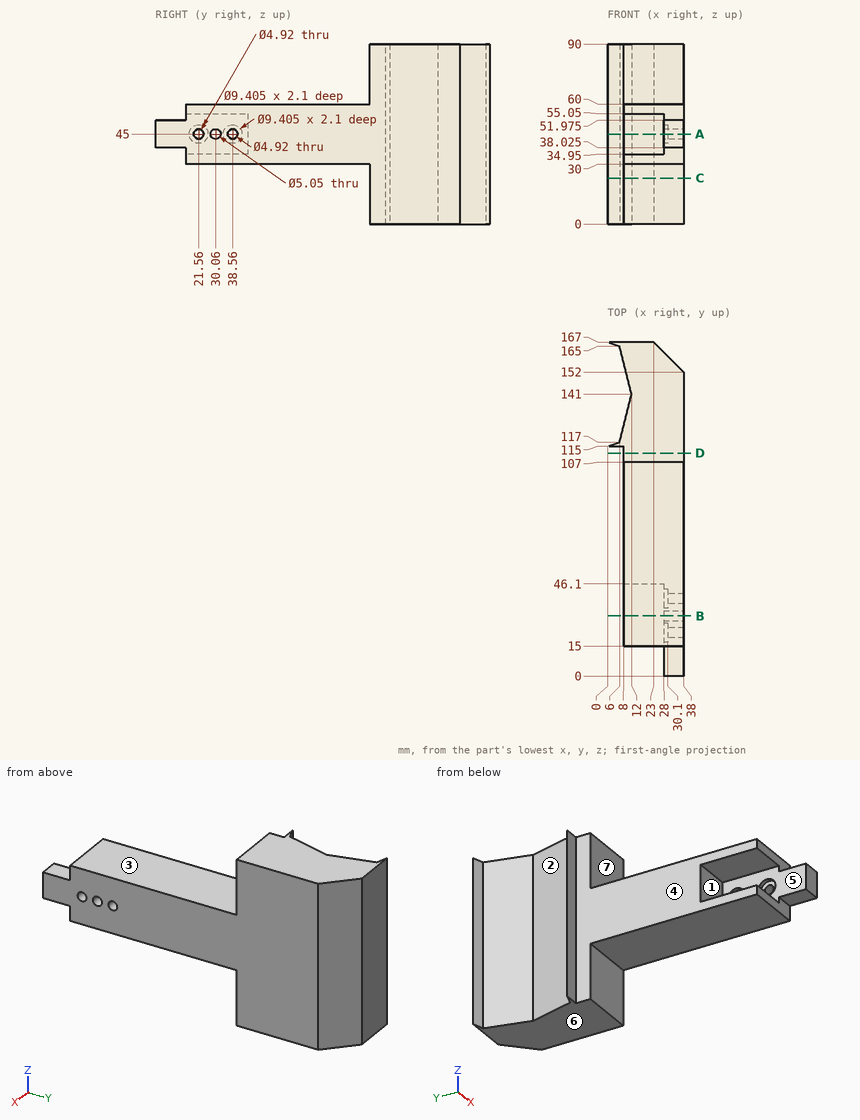
Job drawing, mm, ordinate dimensions from the low corner. One solid piece. A direction names the side the tool comes from. Coordinates: 2 decimals unless noted, no trailing zeros. Loops run counter-clockwise (first coordinate to the right, second up) from the corner with the lowest first, then second, coordinate; pieces in that order, holes last. Notation, with made-up numbers: (87, 42) - (122, 42) arc R22 ccw to (122, 75) - close; hole circle Ø3 at (-11.75, -14). An arc over 180 degrees is marked (long way). Answer as a JSON object with one key per item and string values. Group by question number.
(1) Cut at A-A (z = 45). State how many separate pieces and enclosed holes the cut face has, then the cut area to 3 significant figures.
(2) Cut at C-C (z = 23). Give the cut face in (x, y), then the cut area to 3 significant figures.
(3) Cut at B-B (y = 30.06). Give the cut face in (x, z) (3 decimals), then the cut area to 4 significant figures.
(4) Tool access for the marked faces 1, 2, 3 and 4: list every direction of +Z, -Z, +X, -X, +Y, -Y with a clear straight run to the whole face (end or side of a thin tool).
(5) Flat gauge pins, fed straight in: pin 1 (11 mm diameter, centred on x = 33.5, y = 9, fed in from -Z) (3 decimals); pin 2 (15 mm diameter, centred on x = 25.5, y = 69.5, fed in from +Z); pin 3 (11 mm diameter, centred on x = 33, y = 9, fed in from +Z) (3 decimals). Where does each tip first touch, or does it go through?
(6) Cut at D-D (y = 111.5). Give the cut face in (x, z).
(7) Probe line 1 along Z through (x, y) = (32.25, 21.56); line 2 along Z through (x, y) = (24, 45); line 3 along Y through (x, z) = (34, 45) (3 decimals). List the from-to ranges inside material, lowest first.
(8) Two-plate mould, pull along Z, no slides. Class the marked faces 5, 6 and 7: released by +Z, released by -Z, zero draft, split by the parting line, or undercut.
Geometry says:
{
 "1": {"separate pieces": "4", "enclosed holes": "0", "area": "3,780 mm^2"},
 "2": {"outline": "(0, 115) - (8, 115) - (8, 107) - (38, 107) - (38, 152) - (23, 167) - (0, 167) - (6, 165) - (12, 141) - (6, 117) - close", "area": "1,660 mm^2"},
 "3": {"outline": "(8, 30) - (38, 30) - (38, 42.475) - (28, 42.475) - (28, 34.95) - (8, 34.95) - close; (8, 55.05) - (28, 55.05) - (28, 47.525) - (38, 47.525) - (38, 60) - (8, 60) - close", "area": "447.5 mm^2"},
 "4": {"face 1": "-X, -Y", "face 2": "+Z, -Z, -X", "face 3": "+Z, +X, -X, -Y", "face 4": "+Z, -Z, -X, -Y"},
 "5": {"pin 1": "stops at z = 38.025", "pin 2": "stops at z = 60", "pin 3": "stops at z = 51.975"},
 "6": {"outline": "(8, 0) - (38, 0) - (38, 90) - (8, 90) - close"},
 "7": {"line 1": "z = 30 to 42.54, 47.46 to 60", "line 2": "z = 30 to 34.95, 55.05 to 60", "line 3": "y = 0 to 19.1, 24.02 to 27.535, 32.585 to 36.1, 41.02 to 156"},
 "8": {"face 5": "undercut", "face 6": "released by -Z", "face 7": "zero draft"}
}
